from build123d import *

# Parameters (mm, degrees)
CUT_EXTRUDE1_DEPTH      = 53.974050251
CUT_EXTRUDE1_DEPTH_BACK = 53.974050251
SKETCH2_R               = 1.075
CUT_EXTRUDE2_DEPTH      = 53.974050251
CUT_EXTRUDE2_DEPTH_BACK = 20
SKETCH3_R               = 1.5
CHAMFER1_SIZE           = 0.5


with BuildPart() as part:
    # Sketch1 → Revolve1 (revolve)
    with BuildSketch(Plane(origin=(0, 0, 0), x_dir=(0, 0, -1), z_dir=(1, 0, 0))):
        Polygon((0, 0), (-2.2, 0), (-2.2, 6.001185581), (-5, 10), (-5, 12.5), (-3, 12.5), (-3, 52.5), (0, 52.5), align=None)
    revolve(axis=Axis((0, 52.5, 0), (0, -1, 0)))

    # Sketch2 → Cut-Extrude1 (cut, two sides: drawn at the far end of the back side and taken through both)
    with BuildSketch(Plane(origin=(0, 52.5, 0), x_dir=(1, 0, 0), z_dir=(0, 1, 0)).offset(-CUT_EXTRUDE1_DEPTH_BACK)):
        with Locations(Location((0, 0, 0), (0, 0, 270))):
            Circle(SKETCH2_R)
    extrude(amount=CUT_EXTRUDE1_DEPTH + CUT_EXTRUDE1_DEPTH_BACK, mode=Mode.SUBTRACT)

    # Sketch3 → Cut-Extrude2 (cut, two sides: drawn at the far end of the back side and taken through both)
    with BuildSketch(Plane(origin=(0, 52.5, 0), x_dir=(1, 0, 0), z_dir=(0, 1, 0)).offset(-CUT_EXTRUDE2_DEPTH_BACK)):
        with Locations(Location((0, 0, 0), (0, 0, 270))):
            Circle(SKETCH3_R)
    extrude(amount=CUT_EXTRUDE2_DEPTH + CUT_EXTRUDE2_DEPTH_BACK, mode=Mode.SUBTRACT)

    # Chamfer1
    chamfer1_edges = [part.edges().sort_by_distance(p)[0] for p in [
        (0, 0, -2.2),
    ]]
    chamfer(chamfer1_edges, length=CHAMFER1_SIZE)


solid = part.part
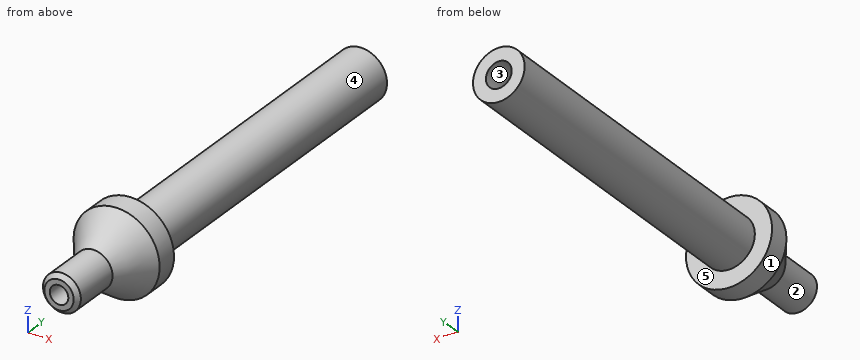
Here's how the part is built. I have some questions about the finished solid (model axes, mm). Face numbers are marked on the shaded views. A direction names the side the tool comes from. Round coordinates to 2 decimals unless told otherwise and drop trailing zeros. Loops run counter-clockwise (first coordinate to the right, second up) from the corner with the lowest first, then second, coordinate; pieces in that order, holes last. Notation, with made-up numbers: M 38.5,-20.75 L 56.5,-20.75 A19 ccw 56.5,7.25 Z; hole C 76,65 d9. An arc over 180 degrees is marked long. Write each question's results on one line, items separated by ' | '. Start each with the question number.
(1) I want a section at D-D (y = 17.5). Please give me the cut outline in (x, z) (3 decimals).
(2) Thinking about a two-plate mould opening in X: for the marked faces 3, 4 and 5, which applies, pulls with the +X half, pulls with the -X half, needs draft (parallel to the pull), parting line crosses it, or undercut?
(3) I want a section at B-B (z = 0). Please give me the cut outline in (x, y) (3 decimals), then the cut area to 3 significant figures.
(4) Will these pins go through, and if not, where does the flat tip stop? P1, Ø3, axis at x = -3, y = 44.5, coming from the +Z side; P2, Ø6, axis at x = 1.5, y = 37.5, coming from the -Z side; P3, Ø6, axis at y = 26, z = 1.5, coming from the +X side.
(5) If I drill on probe 1 along Z at (x, y) = (0, 41.75); probe 2 along X at (y, z) = (20.5, 0) (3 decimals), over which ranges is the centre line in solid material (lowest first)? Write a range as from..to.
(6) I want a section at A-A (x = 0). Please give me the cut outline in (y, z) (3 decimals).
(7) I want a section at C-C (y = 11). Please give me the cut outline in (x, z) (3 decimals), then the cut area to 3 significant figures.
(8) On a 3-axis mill with a long thin cutter (end or side, diameter ignored), from which of +Z, -Z, +X, -X, +Y, -Y can I reach the whole of each face in a straight line? I mean the marked faces 1 and 2. Say none if no direction works.
Solved:
1) outline: C 0,0 d6; hole C 0,0 d2.15
2) face 3: undercut | face 4: parting line crosses it | face 5: needs draft
3) outline: M -5,10 L -2.2,6.001 L -2.2,0.5 L -1.7,0 L -1.075,0 L -1.075,32.5 L -1.5,32.5 L -1.5,52.5 L -3,52.5 L -3,12.5 L -5,12.5 Z; M 1.075,0 L 1.7,0 L 2.2,0.5 L 2.2,6.001 L 5,10 L 5,12.5 L 3,12.5 L 3,52.5 L 1.5,52.5 L 1.5,32.5 L 1.075,32.5 Z | area: 190 mm²
4) P1: stops at z = 2.6 | P2: stops at z = -3 | P3: stops at x = 3
5) probe 1: z = -3..-1.5, 1.5..3 | probe 2: x = -3..-1.075, 1.075..3
6) outline: M 0,-1.7 L 0.5,-2.2 L 6.001,-2.2 L 10,-5 L 12.5,-5 L 12.5,-3 L 52.5,-3 L 52.5,-1.5 L 32.5,-1.5 L 32.5,-1.075 L 0,-1.075 Z; M 0,1.075 L 32.5,1.075 L 32.5,1.5 L 52.5,1.5 L 52.5,3 L 12.5,3 L 12.5,5 L 10,5 L 6.001,2.2 L 0.5,2.2 L 0,1.7 Z
7) outline: C 0,0 d10; hole C 0,0 d2.15 | area: 74.9 mm²
8) face 1: +Y, -Y | face 2: -Y
